Input: part model. Units: mm. Frame: model coordinates. A direction names the side the tool comes from. Give positions to 0.01 mm unless a question says otherwise; leave off trailing zeros. Write each loop counter-clockwise with the first axis right and the second up, starting at its lowest first coordinate (ties: lowest second). Pieces come first, ordered by that corner, then holes. Notation, with made-up numbers: (5, -15.5) -> (35, -15.5) arc R16 ccw to (35, -0.5) -> close; hole circle Ø7 at (3, -25). An arc over 180 degrees is marked (long way). Answer as a JSON object with one key per item and string values. Group by question number.
Autodesk Inventor part; units mm, degrees
ref_plane "YZ Plane" through (0, 0, 0) normal (1, 0, 0) x (0, 1, 0)
ref_plane "XZ Plane" through (0, 0, 0) normal (0, 1, 0) x (-1, 0, 0)
ref_plane "XY Plane" through (0, 0, 0) normal (0, 0, 1) x (1, 0, 0)
sketch "Эскиз24" plane through (0, 0, 0) normal (0, 1, 0) x (1, 0, 0)
  line L0 (0, 0) -> (24.5, 0)
  line L1 (24.5, 0) -> (24.5, 17)
  line L2 (24.5, 17) -> (0, 17)
  line L3 (0, 17) -> (0, 0)
  dimension "d124" = 24.5
  dimension "d125" = 17
extrude "Выдавливание17" add sketch "Эскиз24" along normal blind 4.5
sketch "Эскиз25" plane through (0, 4.5, 0) normal (0, 1, 0) x (1, 0, 0)
  line L0 (24.5, 1) -> (7, 1)
  line L1 (7, 1) -> (7, 16)
  line L2 (7, 16) -> (24.5, 16)
  line L3 (24.5, 16) -> (24.5, 1)
  line L4 (24.5, 0) -> (24.5, 17)
  line L5 (0, 17) -> (0, 0)
  point P0 (24.5, 8.5)
  dimension "d128" = 15
  dimension "d129" = 17.5
extrude "Выдавливание18" cut sketch "Эскиз25" against normal blind 3.5
sketch "Эскиз26" plane through (0, 4.5, 0) normal (0, 1, 0) x (1, 0, 0)
  line L0 (7, 1) -> (7, 16)
  line L1 (2, 5.5) -> (7, 5.5)
  line L2 (7, 5.5) -> (7, 11.5)
  line L3 (7, 11.5) -> (2, 11.5)
  line L4 (2, 11.5) -> (2, 5.5)
  line L5 (7, 1) -> (7, 16)
  point P0 (0, 0)
  point P1 (7, 8.5)
  dimension "d133" = 5
  dimension "d134" = 6
extrude "Выдавливание19" cut sketch "Эскиз26" against normal blind 3
fillet "Сопряжение8" radius 3 2 edges at (4.5, 1.5, -11.5) (4.5, 1.5, -5.5)
sketch "Эскиз27" plane through (0, 4.5, 0) normal (0, 1, 0) x (1, 0, 0)
  line L0 (0, 6.5) -> (2, 6.5)
  line L1 (2, 6.5) -> (2, 10.5)
  line L2 (2, 10.5) -> (0, 10.5)
  line L3 (0, 10.5) -> (0, 6.5)
  line L4 (2, 5.5) -> (2, 11.5)
  line L5 (0, 17) -> (0, 0)
  point P0 (2, 8.5)
  dimension "d138" = 4
extrude "Выдавливание20" cut sketch "Эскиз27" against normal blind 2
fillet "Сопряжение9" radius 2 2 edges at (1, 2.5, -10.5) (1, 2.5, -6.5)
sketch "Эскиз21" plane through (20, 0, 0.1742) normal (1, 0, 0) x (0, 0, -1)
  line L0 (0.1742, 0) -> (-5.0258, 0)
  line L1 (0.1742, 0) -> (0.1742, 25)
  line L2 (-5.0258, 0) -> (-8.7758, -17.85)
  line L3 (0.1742, 0) -> (-3.5758, -17.85)
  line L4 (-8.7758, -17.85) -> (-3.5758, -17.85)
  dimension "d103" = 17.85
  dimension "d104" = 8.95
sketch "Эскиз22" plane through (20, -17.85, 3.75) normal (0, -1, 0) x (1, 0, 0)
  line L0 (0, 0) -> (-9.1, 0)
  line L1 (-9.1, 0) -> (-9.1, 17.3)
  line L2 (-9.1, 17.3) -> (0, 17.3)
  line L3 (0, 17.3) -> (0, 0)
  line L4 (0, 5.2) -> (-9.1, 5.2)
  line L5 (0, 0) -> (-9.1, 0)
  line L6 (0, 5.2) -> (0, 0)
  line L7 (0, 0) -> (-9.1, 0)
  line L8 (-9.1, 0) -> (-9.1, 5.2)
  line L9 (0, 5.2) -> (-9.1, 5.2)
  point P0 (-20, -3.75)
  point P1 (0, -7.9181)
  point P2 (-9.1, -7.9181)
  point P3 (-9.1, 0)
  point P4 (-9.1, -7.9181)
  point P5 (0, -7.9181)
  point P6 (0, 0)
  point P7 (0, 4.1819)
  point P8 (-9.1, 4.1819)
  dimension "d122" = 12.1
sketch "Эскиз23" plane through (40.15, -13.85, 3.75) normal (0, 1, 0) x (1, 0, 0)
  line L0 (-9.1, -17.3) -> (0, -17.3)
  line L1 (-4.55, -17.3) -> (-4.55, -12.6)
  point P0 (-40.15, 3.75)
  dimension "d118" = 4.7
properties part number "Крепление ультрасоника заднее"
1. Mould query, pull axis Z, two halves, no side actions, for faces 1 (the face through (16, 1, -9)), 2 (the face through (12, 0, -9)), 3 (the face through (12, 2, 0)). Classes: pulls with the +Z half, pulls with the -Z half, needs draft (parallel to the pull), parting line crosses it, or undercut.
2. Section C-C (z = -13). Return the cut outline in (x, y).
3. Section D-D (y = 1.95). Return the cut outline in (x, z), plus the area to 3 significant figures.
4. Section B-B (y = 3.75). Return the cut outline in (x, z).
5. Reachability of faces 4 (the face through (12, 2, -17)), 5 (the face through (1.01, 3.1, -7.07)), 6 (the face through (4.54, 2.4, -6.36)) from +Z, -Z, +X, -X, +Y, -Y: full face, straight path, thin tool, end or side. Return the list, or none.
6. Contact query for flat-ended pins moving along their axis: pin 1 Ø0.9 at (y, z) = (2.5, -8) entering from +X; pin 2 Ø6 at (x, z) = (12, -8) entering from +Y. Output: stop coordinate, or through.
7. Line query: line 1 (Z direction, x = 17.5, y = 3.3); line 2 (Y direction, x = 20.25, z = -7); line 3 (X direction, y = 1.3, z = -12.75). Output: solid intervals per line, ascending.
8. Section A-A (x = 11.5). Return the cut outline in (y, z), plus the area to 3 significant figures.
Working result:
{
 "1": {"face 1": "undercut", "face 2": "needs draft", "face 3": "pulls with the +Z half"},
 "2": {"outline": "(0, 0) -> (24.5, 0) -> (24.5, 1) -> (7, 1) -> (7, 4.5) -> (0, 4.5) -> close"},
 "3": {"outline": "(0, -17) -> (24.5, -17) -> (24.5, -16) -> (7, -16) -> (7, -10.08) -> (2, -10.08) -> (2, -6.92) -> (7, -6.92) -> (7, -1) -> (24.5, -1) -> (24.5, 0) -> (0, 0) -> close", "area": "138 mm^2"},
 "4": {"outline": "(0, -17) -> (24.5, -17) -> (24.5, -16) -> (7, -16) -> (7, -11.4) -> (2, -11.4) -> (2, -10.35) -> (0, -10.35) -> close; (0, -6.65) -> (2, -6.65) -> (2, -5.6) -> (7, -5.6) -> (7, -1) -> (24.5, -1) -> (24.5, 0) -> (0, 0) -> close"},
 "5": {"face 4": "-Z, +X, -X, +Y, -Y", "face 5": "+X, -X, +Y", "face 6": "+X, +Y"},
 "6": {"pin 1": "stops at x = 2", "pin 2": "stops at y = 1"},
 "7": {"line 1": "z = -17 to -16, -1 to 0", "line 2": "y = 0 to 1", "line 3": "x = 0 to 7"},
 "8": {"outline": "(0, -17) -> (4.5, -17) -> (4.5, -16) -> (1, -16) -> (1, -1) -> (4.5, -1) -> (4.5, 0) -> (0, 0) -> close", "area": "24.0 mm^2"}
}
